Verification items for this drawing (mm, ordinates from the low corner). Round coordinates to 2 decimals unless told otherwise and drop trailing zeros. Loops run counter-clockwise (first coordinate to the right, second up) from the corner with the lowest first, then second, coordinate; pieces in that order, holes last. Notation, with made-up numbers: M -27,-7 L 4,-7 A26 cw 4,10 Z; hole C 82.5,25 d1. An arc over 180 degrees is marked long. Answer as CSV lines item,"result".
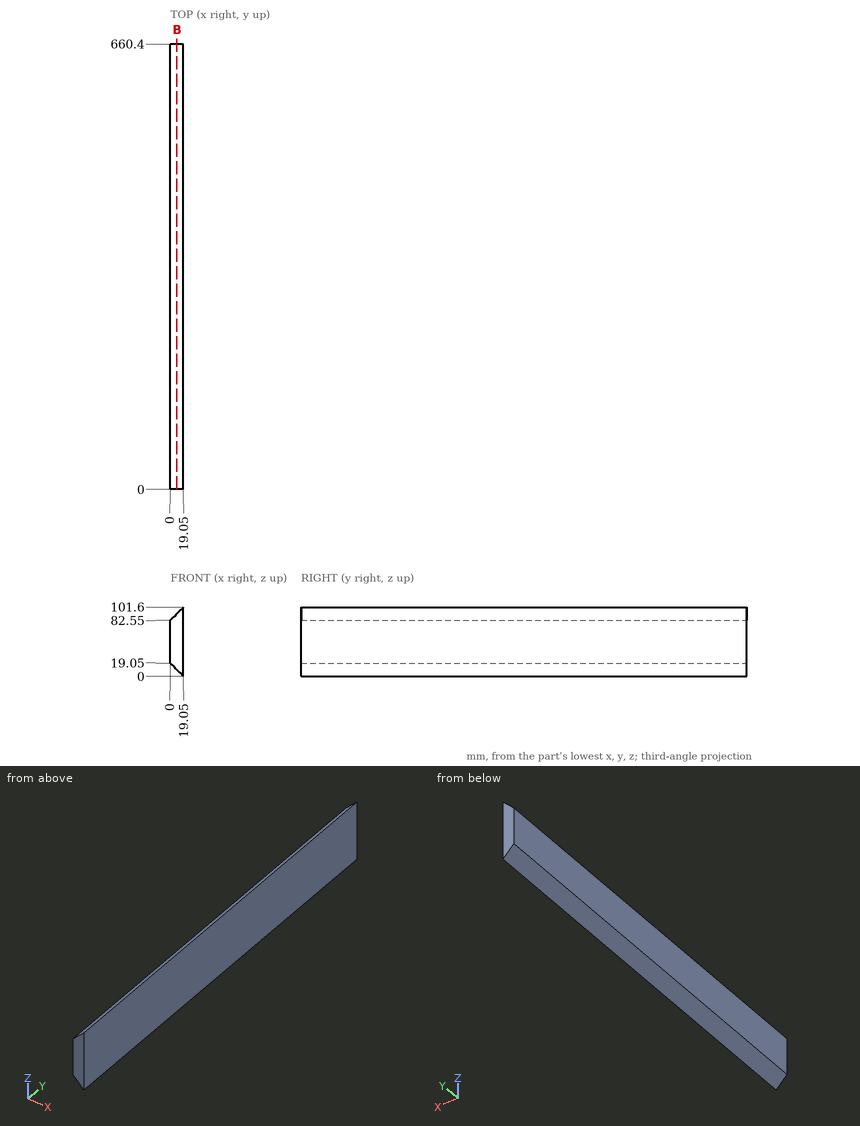
1) Section check B-B (x = 9.75). Record the cut outline in (y, z).
Here are the results:
outline,"M 0,9.3 L 660.4,9.3 L 660.4,92.3 L 0,92.3 Z"
2) Go/stop test with flat-tipped pins: pin 1 (8 mm diameter, centred on x = 14.5, y = 399, fed in from -Z); pin 2 (6 mm diameter, centred on x = 15.5, y = 305.5, fed in from +Z); pin 3 (6 mm diameter, centred on x = 16, y = 412, fed in from +Z). Record where each tip stops, or that it passes through.
Here are the results:
pin 1,"stops at z = 0.55"
pin 2,"stops at z = 101.05"
pin 3,"stops at z = 101.55"
3) Material ranges on probe 1 along Z at (x, y) = (6.75, 327.5); probe 2 along Z at (x, y) = (13.5, 287); probe 3 along X at (y, z) = (364, 93), recorded low to high.
Here are the results:
probe 1,"z = 12.3 to 89.3"
probe 2,"z = 5.55 to 96.05"
probe 3,"x = 10.45 to 19.05"
